Check sheet for the modelled part. Datum: model origin and axes. Units: mm. Face numbers are marked on the shaded views. Coordinates: 2 decimals unless noted, no trailing zeros. Loops run counter-clockwise (first coordinate to the right, second up) from the corner with the lowest first, then second, coordinate; pieces in that order, holes last. Notation, with made-up numbers: (34.25, 9.25) - (72.25, 9.25) arc R8 ccw to (72.25, 20.25) - close; hole circle Ø10 at (60, -20.75). An arc over 180 degrees is marked (long way). Write each question's results on one line, items separated by ' | '. Start each with the question number.
1. Draft check along Z on the marked faces 1 and 2. Enter one of: released by +Z, released by -Z, zero draft, split by the parting line, or undercut.
2. Cross-section at C-C (y = 2.45). Record the cut outline in (x, z), and give its area (3 significant figures).
3. Cross-section at B-B (z = -10). Record the cut outline in (x, y).
4. Cross-section at D-D (x = 10). Record the cut outline in (y, z).
5. Cross-section at A-A (x = -10). Record the cut outline in (y, z).
6. Thickness scan on line 1 (Z direction, x = -10, y = 2.4); line 2 (X direction, y = 1.7, z = -10); line 3 (Z direction, x = -9, y = 3.6). Record the ranges inside material, lowest first. Write a range as [from, to].
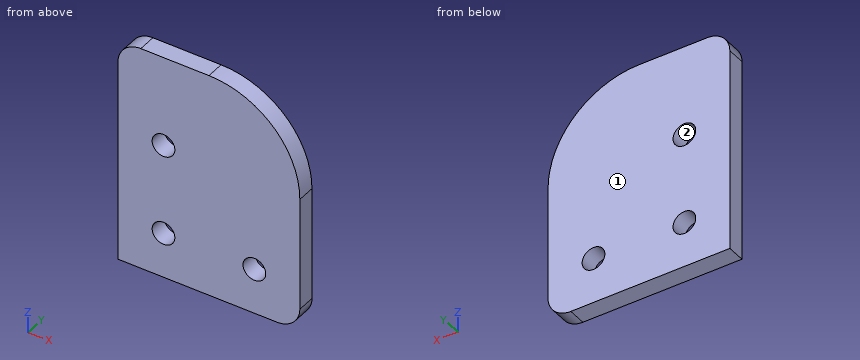
```python
from build123d import *

# Parameters (mm, degrees)
SKETCH1_R           = 2.5
BOSS_EXTRUDE1_DEPTH = 4
FILLET1_R           = 5


with BuildPart() as part:
    # Sketch1 → Boss-Extrude1 (new body)
    with BuildSketch(Plane(origin=(0, 0, 0), x_dir=(1, 0, 0), z_dir=(0, 1, 0))):
        with BuildLine():
            Line((-20, 20), (20, 20))
            Line((20, 20), (20, -10))
            ThreePointArc((20, -10), (14.142135624, -24.142135624), (0, -30))
            Line((0, -30), (-20, -30))
            Line((-20, -30), (-20, 20))
        make_face()
        with Locations((-10, 10)):
            Circle(SKETCH1_R, mode=Mode.SUBTRACT)
        with Locations((10, 10)):
            Circle(SKETCH1_R, mode=Mode.SUBTRACT)
        with Locations((-10, -10)):
            Circle(SKETCH1_R, mode=Mode.SUBTRACT)
    extrude(amount=BOSS_EXTRUDE1_DEPTH)

    # Fillet1
    fillet1_edges = [part.edges().sort_by_distance(p)[0] for p in [
        (20, 2, -20),
        (-20, 2, 30),
    ]]
    fillet(fillet1_edges, radius=FILLET1_R)


solid = part.part
```
Established:
1) face 1: zero draft | face 2: undercut
2) outline: (-20, -20) - (15, -20) arc R5 ccw to (20, -15) - (20, 10) arc R20 ccw to (0, 30) - (-15, 30) arc R5 ccw to (-20, 25) - close; hole circle Ø5 at (-10, -10); hole circle Ø5 at (-10, 10); hole circle Ø5 at (10, -10) | area: 1,840 mm^2
3) outline: (-20, 0) - (-12.5, 0) - (-12.5, 4) - (-20, 4) - close; (-7.5, 0) - (7.5, 0) - (7.5, 4) - (-7.5, 4) - close; (12.5, 0) - (20, 0) - (20, 4) - (12.5, 4) - close
4) outline: (0, -20) - (4, -20) - (4, -12.5) - (0, -12.5) - close; (0, -7.5) - (4, -7.5) - (4, 27.32) - (0, 27.32) - close
5) outline: (0, -20) - (4, -20) - (4, -12.5) - (0, -12.5) - close; (0, -7.5) - (4, -7.5) - (4, 7.5) - (0, 7.5) - close; (0, 12.5) - (4, 12.5) - (4, 30) - (0, 30) - close
6) line 1: [-20, -12.5], [-7.5, 7.5], [12.5, 30] | line 2: [-20, -12.5], [-7.5, 7.5], [12.5, 20] | line 3: [-20, -12.29], [-7.71, 7.71], [12.29, 30]
